from build123d import *

# Parameters (mm, degrees)
CROQUIS1_W                                     = 23
CROQUIS1_H                                     = 14
CROQUIS1_R                                     = 5.1
SALIENTE_EXTRUIR1_DEPTH                        = 30
PERFORADOR_PARA_ROSCAR_PARA_MACHO_DE_ROS_D     = 2.5
PERFORADOR_PARA_ROSCAR_PARA_MACHO_DE_ROS_DEPTH = 12
PERFORADOR_PARA_ROSCAR_PARA_MACHO_DE_ROS_TIP   = 0.751075774


with BuildPart() as part:
    # Croquis1 → Saliente-Extruir1 (new body)
    with BuildSketch(Plane.XY):
        with Locations((11.5, 7)):
            Rectangle(CROQUIS1_W, CROQUIS1_H)
        with Locations((11.5, 7)):
            Circle(CROQUIS1_R, mode=Mode.SUBTRACT)
    extrude(amount=SALIENTE_EXTRUIR1_DEPTH)

    # Perforador para roscar para macho de roscar para M31
    with Locations(Plane.XY.offset(30)):
        with Locations((3.5, 7), (19.5, 7)):
            Hole(PERFORADOR_PARA_ROSCAR_PARA_MACHO_DE_ROS_D / 2, depth=PERFORADOR_PARA_ROSCAR_PARA_MACHO_DE_ROS_DEPTH)
            with Locations((0, 0, -(PERFORADOR_PARA_ROSCAR_PARA_MACHO_DE_ROS_DEPTH + PERFORADOR_PARA_ROSCAR_PARA_MACHO_DE_ROS_TIP / 2))):  # 118° drill point
                Cone(0, PERFORADOR_PARA_ROSCAR_PARA_MACHO_DE_ROS_D / 2, PERFORADOR_PARA_ROSCAR_PARA_MACHO_DE_ROS_TIP, mode=Mode.SUBTRACT)


solid = part.part
Input: part model. Units: mm. Frame: model coordinates. A direction names the side the tool comes from. Coordinates: 2 decimals unless noted, no trailing zeros. Order: outer loops, then holes, each group sorted by start corner. A loop starts at its lowest first (then second) coordinate and runs counter-clockwise, first axis right, second up. Notation, with made-up numbers: M 78.5,74 L 89.5,74 A20 ccw 89.5,78 Z; hole C 19,58 d3. An arc over 180 degrees is marked long. Write item = value, one per line. Start each with the question number.
(1) First-contact query: P1, Ø2, axis at x = 19.5, y = 7, coming from the +Z side. Flat tip, straight axial feed; report the tip coordinate or a pass-through.
(2) Section C-C on z = 22.75. Output: boundary loops of the cut face in (x, y), and give its area (3 significant figures).
(3) Section A-A on x = 11.5. Output: boundary loops of the cut face in (y, z), and give its area (3 significant figures).
(4) Reachability of faces 5 (the flat face through (11, 0, 15)), 6 (the cylindrical face through (2.923, 5.891, 23.916)) from +Z, -Z, +X, -X, +Y, -Y: full face, straight path, thin tool, end or side. Return the list, or none.
(5) Section D-D on z = 5.5. Output: boundary loops of the cut face in (x, y).
(6) Pull-direction query (X, two-part tool) for faces 1 (the flat face through (0, 7, 15)), 2 (the conical face through (19.7, 6.92, 17.38)), 3 (the cylindrical face through (16.364, 8.532, 14.79)), 4 (the flat face through (6, 7, 30)); classes: released by +X, released by -X, zero draft, split by the parting line, or undercut.
(7) Section B-B on y = 11.5. Output: boundary loops of the cut face in (x, z).
(8) Line query: line 1 along Y through (x, z) = (11.75, 14.75); line 2 along Y through (x, z) = (3.5, 23.5); line 3 along X through (y, z) = (4.5, 26.75). Output: solid intervals per line, ascending. Write a range as [from, to].
Result set:
q1.P1 = 17.85
q2.outline = M 0,0 L 23,0 L 23,14 L 0,14 Z; hole C 3.5,7 d2.5; hole C 11.5,7 d10.2; hole C 19.5,7 d2.5
q2.area = 230 mm²
q3.outline = M 0,0 L 1.9,0 L 1.9,30 L 0,30 Z; M 12.1,0 L 14,0 L 14,30 L 12.1,30 Z
q3.area = 114 mm²
q4.face_5 = +Z, -Z, +X, -X, -Y
q4.face_6 = +Z
q5.outline = M 0,0 L 23,0 L 23,14 L 0,14 Z; hole C 11.5,7 d10.2
q6.face_1 = released by -X
q6.face_2 = undercut
q6.face_3 = undercut
q6.face_4 = zero draft
q7.outline = M 0,0 L 9.1,0 L 9.1,30 L 0,30 Z; M 13.9,0 L 23,0 L 23,30 L 13.9,30 Z
q8.line_1 = [0, 1.91], [12.09, 14]
q8.line_2 = [0, 5.75], [8.25, 14]
q8.line_3 = [0, 7.05], [15.95, 23]
